from build123d import *

# Parameters (mm, degrees)
SKETCH_1_R          = 1.95
SKETCH_1_R_2        = 14
EXTRUDE_1_DEPTH     = 5
SKETCH_2_R          = 1.95
CUT_EXTRUDE_1_DEPTH = 40.6408375
FILLET_1_R          = 2


with BuildPart() as part:
    # 草图1 → 凸台-拉伸1 (new body)
    with BuildSketch(Plane.XY):
        with BuildLine():
            Line((-20.668149566, 3.718547232), (-24.575680979, -18))
            Line((-24.575680979, -18), (-24.575680979, -30))
            Line((-24.575680979, -30), (25.424319021, -30))
            Line((25.424319021, -30), (25.424319021, -18))
            Line((25.424319021, -18), (20.516756247, 4.479142005))
            ThreePointArc((20.516756247, 4.479142005), (-0.387757768, 20.996419788), (-20.668149566, 3.718547232))
        make_face()
        with Locations((0, 17.5)):
            Circle(SKETCH_1_R, mode=Mode.SUBTRACT)
        with Locations((17.5, 0)):
            Circle(SKETCH_1_R, mode=Mode.SUBTRACT)
        with Locations((0, -17.5)):
            Circle(SKETCH_1_R, mode=Mode.SUBTRACT)
        with Locations((-17.5, 0)):
            Circle(SKETCH_1_R, mode=Mode.SUBTRACT)
        Circle(SKETCH_1_R_2, mode=Mode.SUBTRACT)
    extrude(amount=EXTRUDE_1_DEPTH)

    # 草图2 → 切除-拉伸1 (cut, through all)
    with BuildSketch(Plane.XY.offset(5)):
        with Locations((19.424319021, -24)):
            Circle(SKETCH_2_R)
        with Locations((-18.575680979, -24)):
            Circle(SKETCH_2_R)
    extrude(amount=-CUT_EXTRUDE_1_DEPTH, mode=Mode.SUBTRACT)

    # 圆角1
    fillet_1_edges = [part.edges().sort_by_distance(p)[0] for p in [
        (25.424319021, -18, 2.5),
        (25.424319021, -30, 2.5),
        (-24.575680979, -30, 2.5),
        (-24.575680979, -18, 2.5),
    ]]
    fillet(fillet_1_edges, radius=FILLET_1_R)


solid = part.part
Verification items for the finished model (mm, model axes). Give positions to 0.01 mm unless a question says otherwise; leave off trailing zeros. Write each loop counter-clockwise with the first axis right and the second up, starting at its lowest first coordinate (ties: lowest second). Pieces come first, ordered by that corner, then holes. Notation, with made-up numbers: (24.25, 58) - (50.25, 58) arc R16 ccw to (50.25, 68) - close; hole circle Ø5 at (63.25, 28.5). An arc over 180 degrees is marked (long way). Answer as CSV lines item,"result". Start each with the question number.
1. Sectioned sample at B-B (x = 16.5). Record the boundary of the cut face in (y, z).
2. Depth check by flat-ended pin: pin 1 (3.5 mm diameter, centred on x = -18.58, y = -24, fed in from +Z); pin 2 (2 mm diameter, centred on y = -16.5, z = 3, fed in from -X). Enter the tip coordinate at first touch or a pass-through.
3. Thickness scan on line 1 (Y direction, x = 0, z = 3.5); line 2 (Y direction, x = -17.5, z = 2.65); line 3 (X direction, y = -0.5, z = 4.35). Record the ranges inside material, lowest first.
4. Draft check along X on faces 1 (the face through (0, -15, 0)), 2 (the face through (-19.448, 0.086, 2.465)), 3 (the face through (25.424, -23, 2)), 4 (the face through (15.552, 0.086, 2.465)). Enter one of: pulls with the +X half, pulls with the -X half, needs draft (parallel to the pull), parting line crosses it, or undercut.
5. Sectioned sample at A-A (y = -24). Record the boundary of the cut face in (x, z).
6. Sectioned sample at C-C (z = 3.85). Record the boundary of the cut face in (x, y).
7. Sectioned sample at D-D (x = -17.5). Record the boundary of the cut face in (y, z), then the cut area to 3 significant figures.
Derived:
1,outline,"(-30, 0) - (-1.67, 0) - (-1.67, 5) - (-30, 5) - close; (1.67, 0) - (12.99, 0) - (12.99, 5) - (1.67, 5) - close"
2,pin 1,"through"
2,pin 2,"x = -24.49"
3,line 1,"-30 to -19.45, -15.55 to -14, 14 to 15.55, 19.45 to 21"
3,line 2,"-30 to -25.63, -22.37 to -1.95, 1.95 to 11.61"
3,line 3,"-21.43 to -19.38, -15.62 to -13.99, 13.99 to 15.62, 19.38 to 21.6"
4,face 1,"needs draft"
4,face 2,"undercut"
4,face 3,"pulls with the +X half"
4,face 4,"undercut"
5,outline,"(-24.58, 0) - (-20.53, 0) - (-20.53, 5) - (-24.58, 5) - close; (-16.63, 0) - (17.47, 0) - (17.47, 5) - (-16.63, 5) - close; (21.37, 0) - (25.42, 0) - (25.42, 5) - (21.37, 5) - close"
6,outline,"(-24.58, -28) arc R2 ccw to (-22.58, -30) - (23.42, -30) arc R2 ccw to (25.42, -28) - (25.42, -18.22) arc R2 ccw to (25.38, -17.79) - (20.52, 4.48) arc R21 ccw to (-20.67, 3.72) - (-24.54, -17.82) arc R2 ccw to (-24.58, -18.18) - close; hole circle Ø3.9 at (-18.58, -24); hole circle Ø3.9 at (-17.5, 0); hole circle Ø28 at (0, 0); hole circle Ø3.9 at (0, -17.5); hole circle Ø3.9 at (0, 17.5); hole circle Ø3.9 at (17.5, 0); hole circle Ø3.9 at (19.42, -24)"
7,outline,"(-30, 0) - (-25.63, 0) - (-25.63, 5) - (-30, 5) - close; (-22.37, 0) - (-1.95, 0) - (-1.95, 5) - (-22.37, 5) - close; (1.95, 0) - (11.61, 0) - (11.61, 5) - (1.95, 5) - close"
7,area,"172 mm²"
